The drawing under review shows one solid part. Ordinate dimensions are in mm from its lowest x, y, z. Coordinates: 2 decimals unless noted, no trailing zeros. Loops run counter-clockwise (first coordinate to the right, second up) from the corner with the lowest first, then second, coordinate; pieces in that order, holes last.
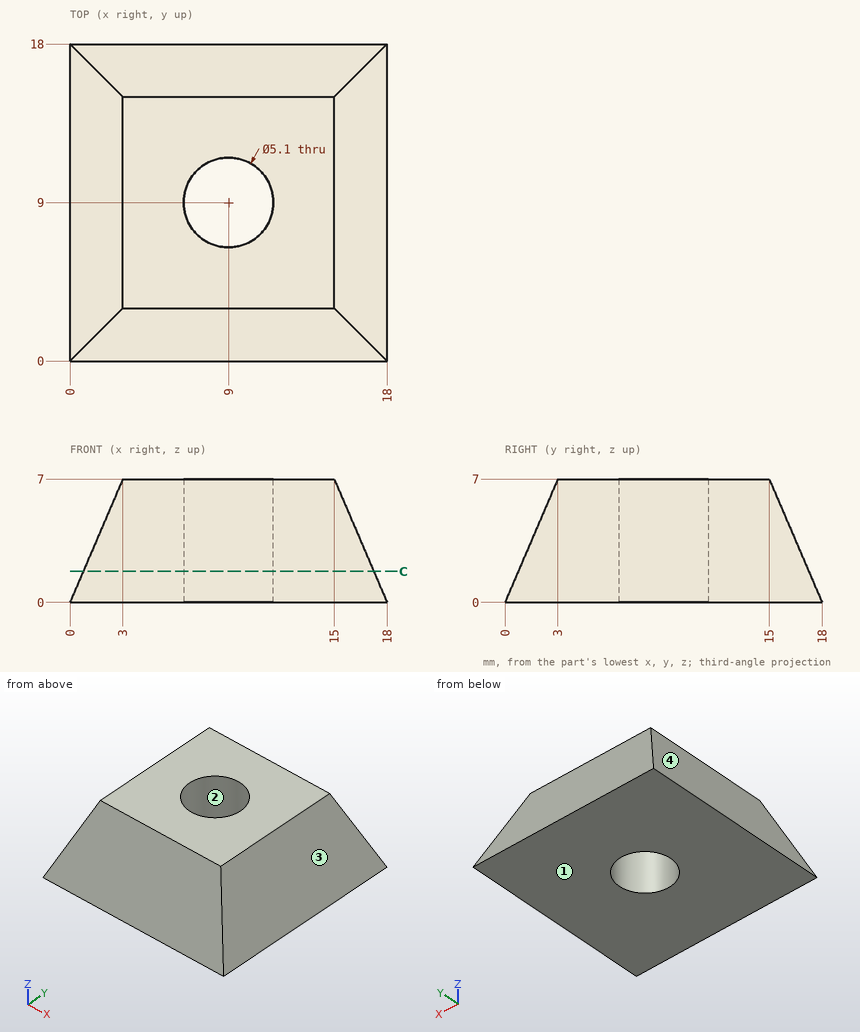
Q1. For line 1 (Y direction, x = 9, z = 5.5); line 2 (X direction, y = 9, z = 1.5); line 3 (X direction, y = 9, z = 5), list the stretches that pass through material, from the lowest coordinate up.
Q2. The part is to be moulded in two halves that separate along X. For the marked faces 1, 2, 3 and 4, say which applies: pulls with the +X half, pulls with the -X half, needs draft (parallel to the pull), parting line crosses it, or undercut.
Q3. Take a section at C-C, the plane z = 1.75. Write out the cut boundary in (x, y).
Q4. Clearance check with flat-ended pins moving along their axes: pin 1 Ø4.5 at (x, y) = (9, 9) entering from -Z; pin 2 Ø2 at (x, z) = (12.5, 4) entering from -Y. State where each tip first meets the part, or that it passes through.
Entries:
1. line 1: y = 2.36 to 6.45, 11.55 to 15.64
1. line 2: x = 0.64 to 6.45, 11.55 to 17.36
1. line 3: x = 2.14 to 6.45, 11.55 to 15.86
2. face 1: needs draft
2. face 2: undercut
2. face 3: pulls with the +X half
2. face 4: pulls with the -X half
3. outline: (0.75, 0.75) - (17.25, 0.75) - (17.25, 17.25) - (0.75, 17.25) - close; hole circle Ø5.1 at (9, 9)
4. pin 1: passes through
4. pin 2: stops at y = 1.29
